```python
from build123d import *

# Parameters (mm, degrees)
SALIENTE_EXTRUIR1_START     = -1.5
SALIENTE_EXTRUIR1_OUTLINE_W = 10
SALIENTE_EXTRUIR1_OUTLINE_H = 2.9
SALIENTE_EXTRUIR1_OUTLINE_R = 1.5
SALIENTE_EXTRUIR1_DEPTH     = 3
CROQUIS2_R                  = 4
CORTAR_EXTRUIR1_DEPTH       = 10


# Read off the part's stored shape, not the designer's step: Saliente-Extruir1
with BuildPart() as part:
    # Saliente-Extruir1 outline → Saliente-Extruir1 (new body)
    with BuildSketch(Plane.XY.offset(SALIENTE_EXTRUIR1_START)):
        with BuildLine():
            ThreePointArc((492.916449572, 98.009593947), (492.452410006, 99.442022929), (491.249851225, 100.348134338))
            ThreePointArc((491.249851225, 100.348134338), (487.916517891, 105.062179546), (491.249851225, 109.776224754))
            ThreePointArc((491.249851225, 109.776224754), (492.452037009, 110.681812922), (492.916439741, 112.113480025))
            Line((492.916439741, 112.113480025), (492.916413331, 149.999679341))
            Line((492.916413331, 149.999679341), (410.416517891, 149.999679341))
            Line((410.416517891, 149.999679341), (410.416517891, 112.133247358))
            ThreePointArc((410.416517891, 112.133247358), (410.875276439, 110.689871685), (412.083184558, 109.776224754))
            ThreePointArc((412.083184558, 109.776224754), (415.416517891, 105.062179546), (412.083184558, 100.348134338))
            ThreePointArc((412.083184558, 100.348134338), (410.875276439, 99.434487407), (410.416517891, 97.991111734))
            Line((410.416517891, 97.991111734), (410.416517891, 52.008362374))
            ThreePointArc((410.416517891, 52.008362374), (410.875276439, 50.564986701), (412.083184558, 49.65133977))
            ThreePointArc((412.083184558, 49.65133977), (415.416517891, 44.937294562), (412.083184558, 40.223249354))
            ThreePointArc((412.083184558, 40.223249354), (410.875276439, 39.309602423), (410.416517891, 37.86622675))
            Line((410.416517891, 37.86622675), (410.416517891, -0.000320659))
            Line((410.416517891, -0.000320659), (492.916517891, -0.000320659))
            Line((492.916517891, -0.000320659), (492.916491488, 37.877716604))
            ThreePointArc((492.916491488, 37.877716604), (492.45443711, 39.314289338), (491.249851225, 40.223249354))
            ThreePointArc((491.249851225, 40.223249354), (487.916517891, 44.937294562), (491.249851225, 49.65133977))
            ThreePointArc((491.249851225, 49.65133977), (492.453865854, 50.559496169), (492.916481647, 51.994900607))
            Line((492.916481647, 51.994900607), (492.916449572, 98.009593947))
        make_face()
        with Locations((421.620579276, 29.951315893)):
            Rectangle(SALIENTE_EXTRUIR1_OUTLINE_W, SALIENTE_EXTRUIR1_OUTLINE_H, mode=Mode.SUBTRACT)
        with Locations((441.347923427, 29.951315893)):
            Circle(SALIENTE_EXTRUIR1_OUTLINE_R, mode=Mode.SUBTRACT)
        with Locations((461.347923427, 29.951315893)):
            Circle(SALIENTE_EXTRUIR1_OUTLINE_R, mode=Mode.SUBTRACT)
        with Locations((481.712351947, 29.951315893)):
            Rectangle(SALIENTE_EXTRUIR1_OUTLINE_W, SALIENTE_EXTRUIR1_OUTLINE_H, mode=Mode.SUBTRACT)
        with Locations((421.620579275, 120.047994692)):
            Rectangle(SALIENTE_EXTRUIR1_OUTLINE_W, SALIENTE_EXTRUIR1_OUTLINE_H, mode=Mode.SUBTRACT)
        with Locations((441.347923427, 120.047994692)):
            Circle(SALIENTE_EXTRUIR1_OUTLINE_R, mode=Mode.SUBTRACT)
        with BuildLine():
            ThreePointArc((448.416504048, 86.999703476), (458.416504048, 96.999703476), (468.416504048, 86.999703476))
            Line((468.416504048, 86.999703476), (468.416487259, 62.999703476))
            ThreePointArc((468.416487259, 62.999703476), (458.416483767, 52.999703476), (448.416487259, 62.999710459))
            Line((448.416487259, 62.999710459), (448.416504048, 86.999703476))
        make_face(mode=Mode.SUBTRACT)
        with Locations((461.347923427, 120.047994692)):
            Circle(SALIENTE_EXTRUIR1_OUTLINE_R, mode=Mode.SUBTRACT)
        with Locations((481.712351947, 120.047994692)):
            Rectangle(SALIENTE_EXTRUIR1_OUTLINE_W, SALIENTE_EXTRUIR1_OUTLINE_H, mode=Mode.SUBTRACT)
    extrude(amount=SALIENTE_EXTRUIR1_DEPTH)

    # Croquis2 → Cortar-Extruir1 (cut)
    with BuildSketch(Plane(origin=(0, 0, -1.5), x_dir=(-1, 0, 0), z_dir=(0, 0, -1))):
        with Locations((-459.916517891, 16.999737054)):
            Circle(CROQUIS2_R)
        with Locations((-459.916517891, 44.999737054)):
            Circle(CROQUIS2_R)
        with Locations((-459.916517891, 111.999737054)):
            Circle(CROQUIS2_R)
        with Locations((-459.916517891, 139.999737054)):
            Circle(CROQUIS2_R)
    extrude(amount=-CORTAR_EXTRUIR1_DEPTH, mode=Mode.SUBTRACT)


solid = part.part
```
Source: CAD feature listing. Evaluate the final solid. Frame: model axes, mm. A direction names the side the tool comes from. Coordinates: 2 decimals unless noted, no trailing zeros. Order: outer loops, then holes, each group sorted by start corner. A loop starts at its lowest first (then second) coordinate and runs counter-clockwise, first axis right, second up. Notation, with made-up numbers: (-11.75, 89.5) - (29.25, 89.5) arc R19 cw to (29.25, 98.5) - close; hole circle Ø8 at (50.5, 15.5). An arc over 180 degrees is marked (long way). One line per item, written item: value.
1) Cut plane C-C on x = 453.5. Output: boundary loops of the cut face in (y, z).
Computed values:
outline: (0, -1.5) - (54.29, -1.5) - (54.29, 1.5) - (0, 1.5) - close; (95.71, -1.5) - (150, -1.5) - (150, 1.5) - (95.71, 1.5) - close
2) Cut plane D-D on z = 0.1. State how many separate pieces and enclosed holes the cut face has, plus the area to 3 significant figures.
Computed values:
separate pieces: 1
enclosed holes: 13
area: 11,100 mm^2
3) Contact query for a flat-ended pin moving along its axis: pin 1 (2.5 mm diameter, centred on x = 441.35, y = 29.95, fed in from -Z). Output: stop coordinate, or through.
Computed values:
pin 1: passes through
4) Cut plane A-A on x = 483. Output: boundary loops of the cut face in (y, z).
Computed values:
outline: (0, -1.5) - (28.5, -1.5) - (28.5, 1.5) - (0, 1.5) - close; (31.4, -1.5) - (118.6, -1.5) - (118.6, 1.5) - (31.4, 1.5) - close; (121.5, -1.5) - (150, -1.5) - (150, 1.5) - (121.5, 1.5) - close
5) Cut plane B-B on y = 84. Output: boundary loops of the cut face in (x, z), plus the area to 4 significant figures.
Computed values:
outline: (410.42, -1.5) - (448.42, -1.5) - (448.42, 1.5) - (410.42, 1.5) - close; (468.42, -1.5) - (492.92, -1.5) - (492.92, 1.5) - (468.42, 1.5) - close
area: 187.5 mm^2
6) Ray query, line 1 (Y direction, x = 424, z = 0); line 2 (X direction, y = 140, z = 1.3); line 3 (Y direction, x = 415, z = -0.5). Return the intervals inside material, ascending. Write a range as [from, to].
Computed values:
line 1: y = [0, 28.5], [31.4, 118.6], [121.5, 150]
line 2: x = [410.42, 455.92], [463.92, 492.92]
line 3: y = [0, 42.94], [46.94, 103.06], [107.06, 150]
7) Mould query, pull axis Y, two halves, no side actions, for faces 1 (the face through (452, 150, 0)), 2 (the face through (482, 121.498, 0)), 3 (the face through (410.417, 131, 0)). Classes: released by +Y, released by -Y, zero draft, split by the parting line, or undercut.
Computed values:
face 1: released by +Y
face 2: undercut
face 3: zero draft
8) Reachability of faces 4 (the face through (458.6, 53, 0)), 5 (the face through (492.917, 19, 0)) from +Z, -Z, +X, -X, +Y, -Y: full face, straight path, thin tool, end or side. Return the list, or none.
Computed values:
face 4: +Z, -Z
face 5: +Z, -Z, +X, +Y, -Y
